Verification items for this drawing (mm, ordinates from the low corner). A direction names the side the tool comes from. Round coordinates to 2 decimals unless told otherwise and drop trailing zeros. Order: outer loops, then holes, each group sorted by start corner. A loop starts at its lowest first (then second) coordinate and runs counter-clockwise, first axis right, second up. Notation, with made-up numbers: M -27.75,37 L 18.25,37 A17 ccw 18.25,62 Z; hole C 32.25,36 d3. An arc over 180 degrees is marked long. Return JSON: item names as keys, results as strings. Group by question number.
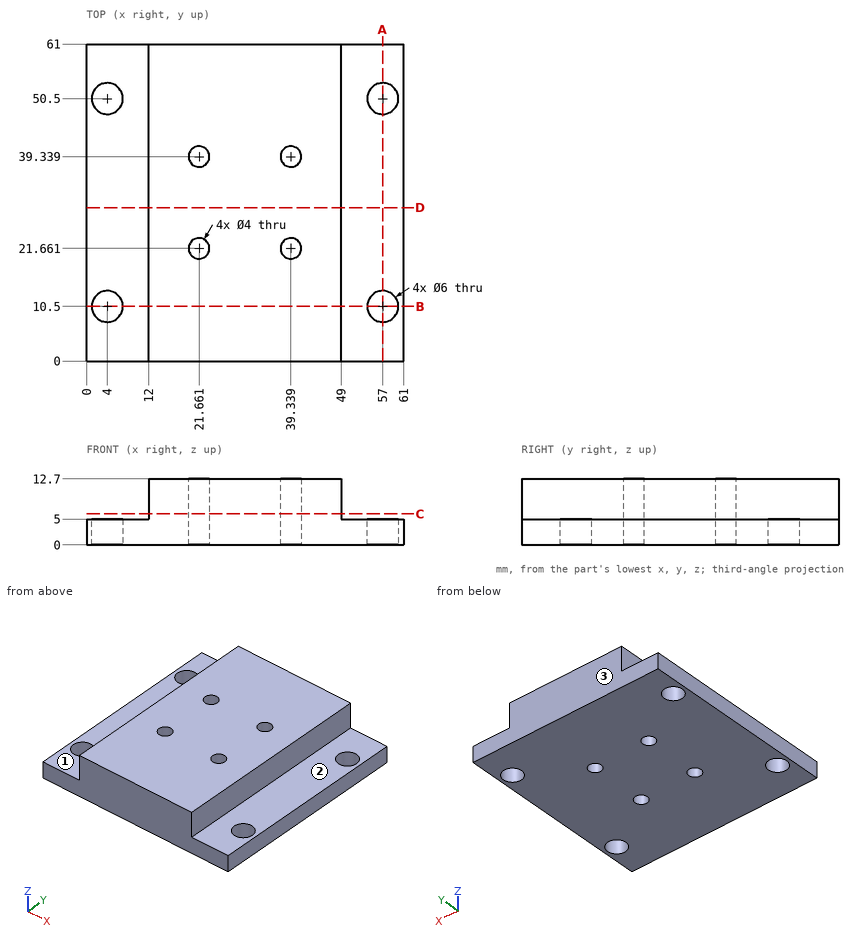
1. Go/stop test with flat-tipped pins: pin 1 (2 mm diameter, centred on y = 25.5, z = 8, fed in from -X); pin 2 (7 mm diameter, centred on x = 4, y = 10.5, fed in from +Z); pin 3 (4 mm diameter, centred on y = 33.5, z = 9.5, fed in from +X). Record where each tip stops, or that it passes through.
2. Access from +Z, -Z, +X, -X, +Y, -Y to the whole of each face (thin tool, end or side, straight path). Record for the marked faces 1, 2 and 3.
3. Cross-section at D-D (y = 29.5). Enter the section's corners in (x, z).
4. Cross-section at C-C (z = 6). Enter the section's corners in (x, y), plus the area to 3 significant figures.
5. Cross-section at B-B (y = 10.5). Enter the section's corners in (x, z), plus the area to 3 significant figures.
6. Thickness scan on line 1 along Y through (x, z) = (21.5, 4.75) (1 decimal); line 2 along Y through (x, z) = (4, 1.35); line 3 along X through (y, z) = (48, 4). Record the ranges inside material, lowest first. Write a range as from..to.
7. Cross-section at A-A (x = 57). Enter the section's corners in (y, z).
Computed:
{
 "1": {"pin 1": "stops at x = 12", "pin 2": "stops at z = 5", "pin 3": "stops at x = 49"},
 "2": {"face 1": "+Z, -X, +Y, -Y", "face 2": "+Z, +X, +Y, -Y", "face 3": "+Z, -Z, +X, -X, +Y"},
 "3": {"outline": "M 0,0 L 61,0 L 61,5 L 49,5 L 49,12.7 L 12,12.7 L 12,5 L 0,5 Z"},
 "4": {"outline": "M 12,0 L 49,0 L 49,61 L 12,61 Z; hole C 21.66,21.66 d4; hole C 21.66,39.34 d4; hole C 39.34,21.66 d4; hole C 39.34,39.34 d4", "area": "2,210 mm²"},
 "5": {"outline": "M 0,0 L 1,0 L 1,5 L 0,5 Z; M 7,0 L 54,0 L 54,5 L 49,5 L 49,12.7 L 12,12.7 L 12,5 L 7,5 Z; M 60,0 L 61,0 L 61,5 L 60,5 Z", "area": "530 mm²"},
 "6": {"line 1": "y = 0..19.7, 23.7..37.3, 41.3..61", "line 2": "y = 0..7.5, 13.5..47.5, 53.5..61", "line 3": "x = 0..2.34, 5.66..55.34, 58.66..61"},
 "7": {"outline": "M 0,0 L 7.5,0 L 7.5,5 L 0,5 Z; M 13.5,0 L 47.5,0 L 47.5,5 L 13.5,5 Z; M 53.5,0 L 61,0 L 61,5 L 53.5,5 Z"}
}
